```python
from build123d import *

# Parameters (mm, degrees)
SKETCH1_R           = 2.05
BOSS_EXTRUDE1_DEPTH = 2
SKETCH3_R           = 0.65
CUT_EXTRUDE1_DEPTH  = 16.490262281
SKETCH4_R           = 0.65
CUT_EXTRUDE2_DEPTH  = 16.490262281
BOSS_EXTRUDE2_DEPTH = 2


with BuildPart() as part:
    # Sketch1 → Boss-Extrude1 (new body)
    with BuildSketch(Plane(origin=(0, 0, 0), x_dir=(1, 0, 0), z_dir=(0, 1, 0))):
        Polygon((-3.5, 6.76929), (-3.5, 0.98071), (3.5, 0.98071), (3.5, 6.76929), (13.78858, 6.76929), (13.78858, -6.76929), (-13.78858, -6.76929), (-13.78858, 6.76929), align=None)
        with Locations(Location((-8.84, 1.81955, 0), (0, 0, 270))):
            Circle(SKETCH1_R, mode=Mode.SUBTRACT)
        with Locations(Location((8.84, 1.81955, 0), (0, 0, 270))):
            Circle(SKETCH1_R, mode=Mode.SUBTRACT)
    extrude(amount=BOSS_EXTRUDE1_DEPTH)

    # Sketch3 → Cut-Extrude1 (cut, through all)
    with BuildSketch(Plane(origin=(0, 2, 0), x_dir=(1, 0, 0), z_dir=(0, 1, 0))):
        with Locations(Location((-0.00858, -1.01929, 0), (0, 0, 270))):
            Circle(SKETCH3_R)
    extrude(amount=-CUT_EXTRUDE1_DEPTH, mode=Mode.SUBTRACT)

    # Sketch4 → Cut-Extrude2 (cut, through all)
    with BuildSketch(Plane(origin=(0, 2, 0), x_dir=(1, 0, 0), z_dir=(0, 1, 0))):
        with Locations((6, -7.01929)):
            Circle(SKETCH4_R)
        with Locations((-6, -7.01929)):
            Circle(SKETCH4_R)
    extrude(amount=-CUT_EXTRUDE2_DEPTH, mode=Mode.SUBTRACT)

    # Sketch5 → Boss-Extrude2 (add)
    with BuildSketch(Plane(origin=(0, 2, 0), x_dir=(1, 0, 0), z_dir=(0, 1, 0))):
        Polygon((-13.78858, -6.76929), (-23.78858, -6.76929), (-23.78858, 16.76929), (-3.5, 16.76929), (-3.5, 6.76929), (-13.78858, 6.76929), align=None)
        Polygon((3.5, 6.76929), (3.5, 16.76929), (23.78858, 16.76929), (23.78858, -6.76929), (13.78858, -6.76929), (13.78858, 6.76929), align=None)
    extrude(amount=-BOSS_EXTRUDE2_DEPTH)


solid = part.part
```
Input: part model. Units: mm. Frame: model coordinates. A direction names the side the tool comes from. Give positions to 0.01 mm unless a question says otherwise; leave off trailing zeros. Order: outer loops, then holes, each group sorted by start corner. A loop starts at its lowest first (then second) coordinate and runs counter-clockwise, first axis right, second up.
1. Line query: probe 1 along X at (y, z) = (0.2, -8); probe 2 along Z at (x, y) = (0, 0.7); probe 3 along X at (y, z) = (1, -1.5). Output: solid intervals per line, ascending.
Computed:
probe 1: x = -23.79 to -3.5, 3.5 to 23.79
probe 2: z = -0.98 to 0.37, 1.67 to 6.77
probe 3: x = -23.79 to -10.86, -6.82 to -3.5, 3.5 to 6.82, 10.86 to 23.79
2. Cut plane B-B (x = -8.84). Return loops of the section in (y, z).
Computed:
outline: (0, -16.77) - (2, -16.77) - (2, -3.87) - (0, -3.87) - close; (0, 0.23) - (2, 0.23) - (2, 6.77) - (0, 6.77) - close
3. Cut plane C-C (y = 1.05). Return loops of the section in (x, z).
Computed:
outline: (-23.79, -16.77) - (-3.5, -16.77) - (-3.5, -0.98) - (3.5, -0.98) - (3.5, -16.77) - (23.79, -16.77) - (23.79, 6.77) - (6.6, 6.77) arc R0.65 cw to (5.4, 6.77) - (-5.4, 6.77) arc R0.65 cw to (-6.6, 6.77) - (-23.79, 6.77) - close; hole circle Ø4.1 at (-8.84, -1.82); hole circle Ø1.3 at (-0.01, 1.02); hole circle Ø4.1 at (8.84, -1.82)
4. Pin query (flat end, axial travel): pin 1 Ø2.5 at (x, z) = (-8.84, -1.82) entering from -Y; pin 2 Ø0.6 at (x, y) = (0.5, 1.5) entering from -Z. Return the tip coordinate at first contact, or that it passes through.
Computed:
pin 1: passes through
pin 2: stops at z = -0.98
5. Cut plane A-A (z = -12.75). Return loops of the section in (x, y).
Computed:
outline: (-23.79, 0) - (-3.5, 0) - (-3.5, 2) - (-23.79, 2) - close; (3.5, 0) - (23.79, 0) - (23.79, 2) - (3.5, 2) - close
6. Draft query along X for faces 3 (the face through (-14, 1, -16.769)), 4 (the face through (-3.5, 1, -9)), 5 (the face through (-23.789, 1, -5)). Return one class per face: released by +X, released by -X, zero draft, split by the parting line, or undercut.
Computed:
face 3: zero draft
face 4: undercut
face 5: released by -X
7. Set-up query: faces 1 (the face through (0, 2, 0)), 2 (the face through (3.5, 1, -9)). Return all of +Z, -Z, +X, -X, +Y, -Y with unobstructed straight access to the full face (end or side cutting, diameter ignored); none if empty.
Computed:
face 1: +Z, -Z, +X, -X, +Y
face 2: -Z, +Y, -Y
